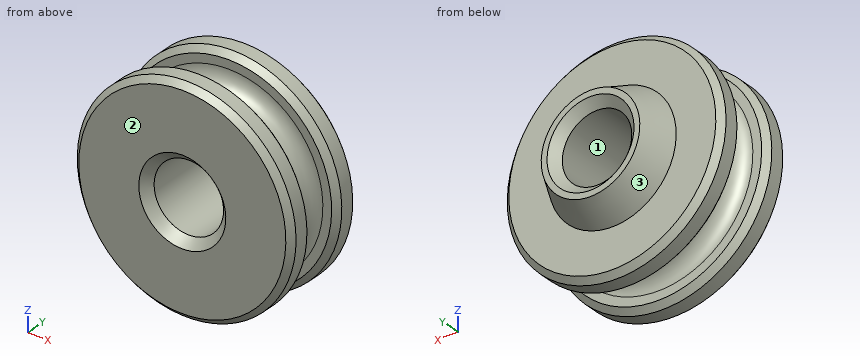
from build123d import *

# Parameters (mm, degrees)
CHAMFER1_SIZE = 0.3
CHAMFER2_SIZE = 0.2


with BuildPart() as part:
    # Sketch1 → Revolve1 (revolve)
    with BuildSketch(Plane(origin=(0, 0, 0), x_dir=(0, 0, -1), z_dir=(1, 0, 0)), mode=Mode.PRIVATE) as revolve1_sk:
        with BuildLine():
            Line((1.191, 2.5), (1.191, -1.5))
            Line((1.191, -1.5), (2.191, -1.5))
            Line((2.191, -1.5), (3.75, -1.5))
            Line((3.75, -1.5), (3.75, -0.6))
            Line((3.75, -0.6), (3.25, -0.6))
            ThreePointArc((3.25, -0.6), (2.65, 0), (3.25, 0.6))
            Line((3.25, 0.6), (3.75, 0.6))
            Line((3.75, 0.6), (3.75, 1.5))
            Line((3.75, 1.5), (2.191, 1.5))
            Line((2.191, 1.5), (1.691, 2.5))
            Line((1.691, 2.5), (1.191, 2.5))
        make_face()
    revolve(revolve1_sk.sketch.rotate(Axis((0, 2.7, 0), (0, -1, 0)), 180), axis=Axis((0, 2.7, 0), (0, -1, 0)))

    # Chamfer1
    chamfer1_edges = [part.edges().sort_by_distance(p)[0] for p in [
        (0, -1.5, -1.191),
        (0, 2.5, -1.191),
    ]]
    chamfer(chamfer1_edges, length=CHAMFER1_SIZE)

    # Chamfer2
    chamfer2_edges = [part.edges().sort_by_distance(p)[0] for p in [
        (0, 1.5, -3.75),
        (0, 0.6, -3.75),
        (0, -0.6, -3.75),
        (0, -1.5, -3.75),
    ]]
    chamfer(chamfer2_edges, length=CHAMFER2_SIZE)


solid = part.part
Can you work these out from the model? Positions are in its coordinate system, mm. Face numbers are marked on the shaded views. Give positions to 0.01 mm unless a question says otherwise; leave off trailing zeros. Loops run counter-clockwise (first coordinate to the right, second up) from the corner with the lowest first, then second, coordinate; pieces in that order, holes last. Notation, with made-up numbers: M -26,-13.5 L 32,-13.5 A13 cw 32,-8.5 Z; hole C -21.5,-21.75 d4. An arc over 180 degrees is marked long. One line per item, written item: value. Start each with the question number.
1) I'm going to push flat-ended pins straight in: pin 1 (1.5 mm diameter, centred on x = -0.5, y = 1, fed in from +Z); pin 2 (1 mm diameter, centred on y = -0.5, z = -2.5, fed in from -X); pin 3 (2.5 mm diameter, centred on x = 0, z = 0, fed in from -Y). Where does each tip first touch, or does it pass through?
2) Thinking about a two-plate mould opening in Z: for the marked faces 1, 2 and 3, which applies, +Z half, -Z half, draft (parallel to the pull), parting line (faces both ways), or undercut?
3) If we section it at C-C, the plane y = -1: Write out the boundary of the cut face in (x, z), and give its area (3 significant figures).
4) If I drill on line 1 (X direction, y = 1.05, z = 0); line 2 (X direction, y = 0.4, z = 0); line 3 (Z direction, x = 1, y = -1.1), over which ranges is the centre line in solid material (lowest first)? Write a range as [from, to].
5) If we section it at D-D, the plane y = 1.4: Write out the boundary of the cut face in (x, z).
Completed:
1. pin 1: stops at z = 3.75
1. pin 2: stops at x = -3.11
1. pin 3: stops at y = -1.26
2. face 1: undercut
2. face 2: draft
2. face 3: parting line
3. outline: C 0,0 d7.5; hole C 0,0 d2.38
3. area: 39.7 mm^2
4. line 1: x = [-3.75, -1.19], [1.19, 3.75]
4. line 2: x = [-2.8, -1.19], [1.19, 2.8]
4. line 3: z = [-3.61, -0.65], [0.65, 3.61]
5. outline: C 0,0 d7.3; hole C 0,0 d2.38
